Work out the finished part from the listing and answer in its coordinate system (mm). A direction names the side the tool comes from. Coordinates: 2 decimals unless noted, no trailing zeros. Write each loop counter-clockwise with the first axis right and the second up, starting at its lowest first coordinate (ties: lowest second). Pieces come first, ordered by that corner, then holes. Notation, with made-up numbers: (77, 51) - (127, 51) arc R17 ccw to (127, 73) - close; hole circle Ø7 at (21.5, -20). An arc over 180 degrees is marked (long way). Use one line per item in the form item = value. Start each with the question number.
Item 1: Determine the mould class of faces 1 (the cylindrical face through (134.437, 0.268, 6.094)), 2 (the flat face through (130, -6, -2)), 3 (the cylindrical face through (135.07, -1.978, 2.579)) for opening direction Y: released by +Y, released by -Y, zero draft, split by the parting line, or undercut.
Item 2: A cutting plane is placed at A-A (z = 0). Write down the section's boundary in (x, y), then the cut area to 3 significant figures.
Item 3: For faces 4 (the flat face through (130, 0, 0)), 5 (the flat face through (0, 0, 0)), determine the directions among +Z, -Z, +X, -X, +Y, -Y from which every point of the face is accessible in a straight line to the end or side of a thin tool.
Item 4: A cutting plane is placed at C-C (x = 54). Write down the section's boundary in (y, z), then the cut area to 3 significant figures.
Item 5: Given pin 1 (2 mm diameter, centred on y = 1.5, z = 1, fed in from +X); pin 2 (4 mm diameter, centred on x = 64.5, z = -4.5, fed in from +Y); pin 3 (1.5 mm diameter, centred on x = 98.5, y = 5, fed in from -Z), each flat-ended and moving along its own axis, determine where each tip first touches the part or whether it passes through.
Item 6: Consider probe 1 along Y at (x, z) = (136, 0); probe 2 along X at (y, z) = (-6.25, 0.5); probe 3 along Z at (x, y) = (133.5, -0.5). Determine where each line is inside the solid, lowest interval first.
from build123d import *

# Parameters (mm, degrees)
IZIM1_W               = 140
IZIM1_H               = 8
KES_EKSTR_ZYON1_START = -10
IZIM2_R               = 8
IZIM2_R_2             = 6.1
KES_EKSTR_ZYON1_DEPTH = 10
IZIM3_R               = 3.25
KES_EKSTR_ZYON2_DEPTH = 10
RADYUS1_R             = 2
RADYUS2_R             = 1


with BuildPart() as part:
    # Çizim1 → Döndür1 (revolve)
    with BuildSketch(Plane.XY, mode=Mode.PRIVATE) as d_nd_r1_sk:
        with Locations((70, 4)):
            Rectangle(IZIM1_W, IZIM1_H)
    revolve(d_nd_r1_sk.sketch.rotate(Axis((0, 0, 0), (1, 0, 0)), 90), axis=Axis((0, 0, 0), (1, 0, 0)))

    # Çizim2 → Kes-Ekstrüzyon1 (cut)
    with BuildSketch(Plane(origin=(140, 0, 0), x_dir=(0, 0, -1), z_dir=(1, 0, 0)).offset(KES_EKSTR_ZYON1_START)):
        with Locations(Location((0, 0, 0), (0, 0, 180))):
            Circle(IZIM2_R)
        Circle(IZIM2_R_2, mode=Mode.SUBTRACT)
    extrude(amount=KES_EKSTR_ZYON1_DEPTH, mode=Mode.SUBTRACT)

    # Çizim3 → Kes-Ekstrüzyon2 (cut)
    with BuildSketch(Plane(origin=(140, 0, 0), x_dir=(0, 0, -1), z_dir=(1, 0, 0))):
        Circle(IZIM3_R)
    extrude(amount=-KES_EKSTR_ZYON2_DEPTH, mode=Mode.SUBTRACT)

    # Radyus1
    radyus1_edges = [part.edges().sort_by_distance(p)[0] for p in [
        (0, 0, -8),
    ]]
    fillet(radyus1_edges, radius=RADYUS1_R)

    # Radyus2
    radyus2_edges = [part.edges().sort_by_distance(p)[0] for p in [
        (130, 0, -8),
        (140, 0, 6.1),
    ]]
    fillet(radyus2_edges, radius=RADYUS2_R)


solid = part.part
Answer:
q1.face_1 = split by the parting line
q1.face_2 = zero draft
q1.face_3 = undercut
q2.outline = (0, -6) arc R2 ccw to (2, -8) - (129, -8) arc R1 ccw to (130, -7) - (130, -6.1) - (139, -6.1) arc R1 ccw to (140, -5.1) - (140, -3.25) - (130, -3.25) - (130, 3.25) - (140, 3.25) - (140, 5.1) arc R1 ccw to (139, 6.1) - (130, 6.1) - (130, 7) arc R1 ccw to (129, 8) - (2, 8) arc R2 ccw to (0, 6) - close
q2.area = 2,130 mm²
q3.face_4 = +X
q3.face_5 = +Z, -Z, -X, +Y, -Y
q4.outline = circle Ø16 at (0, 0)
q4.area = 201 mm²
q5.pin_1 = 130
q5.pin_2 = 7.6
q5.pin_3 = -6.78
q6.probe_1 = -6.1 to -3.25, 3.25 to 6.1
q6.probe_2 = 0.02 to 130
q6.probe_3 = -6.08 to -3.21, 3.21 to 6.08
